from build123d import *

# Parameters (mm, degrees)
SKETCH_2_R          = 2.5
SKETCH_2_R_2        = 4
EXTRUDE_1_DEPTH     = 3
SKETCH_2_3_R        = 4
SKETCH_2_3_R_2      = 2
EXTRUDE_2_DEPTH     = 11.5
SKETCH_6_R          = 2
EXTRUDE_3_DEPTH     = 2.3
FILLET_1_R          = 2
SKETCH_7_R          = 2.5
SKETCH_7_R_2        = 2
CUT_EXTRUDE_2_DEPTH = 2
FILLET_2_R          = 1
CUT_EXTRUDE_3_REACH = 51.374
SKETCH_8_R          = 1.5
CUT_EXTRUDE_4_REACH = 51.374
SKETCH_11_R         = 1.5


with BuildPart() as part:
    # Sketch 2 → Extrude 1 (new body)
    with BuildSketch(Plane.XY):
        Polygon((-41.138288377, 15.425110404), (-41.138288377, 21.570131373), (-25.053133429, 21.570131373), (-20.677655191, 25.94560961), (-13.728698976, 25.94560961), (-8.574109119, 23.757870491), (35.231937864, 23.757870491), (41.138288377, 21.251065018), (41.138288377, -25.94560961), (-41.138288377, -25.94560961), (-41.138288377, -12.020899542), (-33.095710903, -12.020899542), (-33.095710903, 11.403821667), (-37.11699964, 11.403821667), align=None)
        with Locations((10.421946091, 8.532959579)):
            Circle(SKETCH_2_R, mode=Mode.SUBTRACT)
        with Locations((-7.306059133, -18.107570273)):
            Circle(SKETCH_2_R, mode=Mode.SUBTRACT)
        with Locations((25.421946091, 18.532959579)):
            Circle(SKETCH_2_R_2, mode=Mode.SUBTRACT)
        with Locations((-28.314407571, 7.976729123)):
            Circle(SKETCH_2_R_2, mode=Mode.SUBTRACT)
        with Locations((-17, 20.7)):
            Circle(SKETCH_2_R, mode=Mode.SUBTRACT)
        with BuildLine():
            Line((25.543402205, -5.467040421), (31.421946091, -5.467040421))
            ThreePointArc((31.421946091, -5.467040421), (32.129052872, -5.174147202), (32.421946091, -4.467040421))
            Line((32.421946091, -4.467040421), (32.421946091, 1.411503465))
            ThreePointArc((32.421946091, 1.411503465), (32.076213917, 2.167766389), (31.278078869, 2.401100465))
            ThreePointArc((31.278078869, 2.401100465), (26.799843583, 0.155062087), (24.553805205, -4.323173199))
            ThreePointArc((24.553805205, -4.323173199), (24.78713928, -5.121308248), (25.543402205, -5.467040421))
        make_face(mode=Mode.SUBTRACT)
    extrude(amount=EXTRUDE_1_DEPTH)

    # Sketch 2_3 → Extrude 2 (add)
    # profile 1 of 3: a face of its own
    with BuildSketch(Plane.XY):
        with Locations((-28.314407571, 7.976729123)):
            Circle(SKETCH_2_3_R)
        with Locations((-28.314407571, 7.976729123)):
            Circle(SKETCH_2_3_R_2, mode=Mode.SUBTRACT)
    # profile 2 of 3: a face of its own
    with BuildSketch(Plane.XY):
        with Locations((25.421946091, 18.532959579)):
            Circle(SKETCH_2_3_R)
        with Locations((25.421946091, 18.532959579)):
            Circle(SKETCH_2_3_R_2, mode=Mode.SUBTRACT)
    # profile 3 of 3: a face of its own
    with BuildSketch(Plane.XY):
        with BuildLine():
            Line((25.543402205, -5.467040421), (31.421946091, -5.467040421))
            ThreePointArc((31.421946091, -5.467040421), (32.129052872, -5.174147202), (32.421946091, -4.467040421))
            Line((32.421946091, -4.467040421), (32.421946091, 1.411503465))
            ThreePointArc((32.421946091, 1.411503465), (32.076213917, 2.167766389), (31.278078869, 2.401100465))
            ThreePointArc((31.278078869, 2.401100465), (26.799843583, 0.155062087), (24.553805205, -4.323173199))
            ThreePointArc((24.553805205, -4.323173199), (24.78713928, -5.121308248), (25.543402205, -5.467040421))
        make_face()
        with Locations((29.464448227, -2.509542558)):
            Circle(SKETCH_2_3_R_2, mode=Mode.SUBTRACT)
    extrude(amount=EXTRUDE_2_DEPTH)

    # Sketch 6 → Extrude 3 (add, symmetric)
    with BuildSketch(Plane(origin=(1.480786333, -5.526369829, 0), x_dir=(0, 0, 1), z_dir=(-0.25881904510252574, 0.9659258262890671, 0))):
        with Locations(Location((7.25, 26.715994864, 0), (0, 0, 90))):
            Circle(SKETCH_6_R)
    extrude(amount=EXTRUDE_3_DEPTH, both=True)

    # Fillet 1
    fillet_1_edges = [part.edges().sort_by_distance(p)[0] for p in [
        (24.75932029, 3.092229761, 7.25),
    ]]
    fillet(fillet_1_edges, radius=FILLET_1_R)

    # Sketch 7 → Cut-Extrude 2 (cut)
    with BuildSketch(Plane(origin=(1.480786333, -5.526369829, 0), x_dir=(0, 0, 1), z_dir=(-0.25881904510252574, 0.9659258262890671, 0))):
        with Locations((7.25, 26.715994864)):
            Circle(SKETCH_7_R)
        with Locations(Location((7.25, 26.715994864, 0), (0, 0, 270))):
            Circle(SKETCH_7_R_2, mode=Mode.SUBTRACT)
    extrude(amount=-CUT_EXTRUDE_2_DEPTH, mode=Mode.SUBTRACT)

    # Fillet 2
    fillet_2_edges = [part.edges().sort_by_distance(p)[0] for p in [
        (32.421946091, -1.527768478, 3),
        (32.129052872, -5.174147202, 3),
        (21.421946091, 18.532959579, 3),
        (-32.314407571, 7.976729123, 3),
        (28.482674148, -5.467040421, 3),
        (24.78713928, -5.121308248, 3),
        (26.799843583, 0.155062087, 3),
        (32.076213917, 2.167766389, 3),
    ]]
    fillet(fillet_2_edges, radius=FILLET_2_R)

    # Sketch 8 → Cut-Extrude 3 (cut, up to next)
    with BuildSketch(Plane.XY.offset(3), mode=Mode.PRIVATE) as cut_extrude_3_sk1:
        with Locations((-37.138288377, -18.983254576)):
            Circle(SKETCH_8_R)
    cut_extrude_3_tool1 = extrude(cut_extrude_3_sk1.sketch, amount=-CUT_EXTRUDE_3_REACH, mode=Mode.PRIVATE) & part.part
    # Sketch 8 → Cut-Extrude 3 (cut, up to next)
    with BuildSketch(Plane.XY.offset(3), mode=Mode.PRIVATE) as cut_extrude_3_sk2:
        with Locations((-31.138288377, -18.983254576)):
            Circle(SKETCH_8_R)
    cut_extrude_3_tool2 = extrude(cut_extrude_3_sk2.sketch, amount=-CUT_EXTRUDE_3_REACH, mode=Mode.PRIVATE) & part.part
    add(cut_extrude_3_tool1.solids().sort_by_distance((-37.138288, -18.983255, 3))[0], mode=Mode.SUBTRACT)
    add(cut_extrude_3_tool2.solids().sort_by_distance((-31.138288, -18.983255, 3))[0], mode=Mode.SUBTRACT)

    # Sketch 11 → Cut-Extrude 4 (cut, up to next)
    with BuildSketch(Plane.XY.offset(3), mode=Mode.PRIVATE) as cut_extrude_4_sk1:
        with Locations((37.138288377, -18.983254576)):
            Circle(SKETCH_11_R)
    cut_extrude_4_tool1 = extrude(cut_extrude_4_sk1.sketch, amount=-CUT_EXTRUDE_4_REACH, mode=Mode.PRIVATE) & part.part
    # Sketch 11 → Cut-Extrude 4 (cut, up to next)
    with BuildSketch(Plane.XY.offset(3), mode=Mode.PRIVATE) as cut_extrude_4_sk2:
        with Locations((31.138288377, -18.983254576)):
            Circle(SKETCH_11_R)
    cut_extrude_4_tool2 = extrude(cut_extrude_4_sk2.sketch, amount=-CUT_EXTRUDE_4_REACH, mode=Mode.PRIVATE) & part.part
    add(cut_extrude_4_tool1.solids().sort_by_distance((37.138288, -18.983255, 3))[0], mode=Mode.SUBTRACT)
    add(cut_extrude_4_tool2.solids().sort_by_distance((31.138288, -18.983255, 3))[0], mode=Mode.SUBTRACT)


solid = part.part
Read the model definition and answer for the solid it produces. Units are mm, in the model's axes. A direction names the side the tool comes from. Coordinates: 2 decimals unless noted, no trailing zeros. Write each loop counter-clockwise with the first axis right and the second up, starting at its lowest first coordinate (ties: lowest second). Pieces come first, ordered by that corner, then holes. Notation, with made-up numbers: M 17.5,87.25 L 73.5,87.25 A26 cw 73.5,107.25 Z; hole C 21.25,73.25 d8. An arc over 180 degrees is marked long. Use a Markdown table: item, result.
Q1. Determine the mould class of faces 4 (the face through (32.524, -19.558, 1.521)), 5 (the face through (-33, 21.57, 1)), 6 (the face through (27.3, 15, 7.7)) for opening direction X: released by +X, released by -X, zero draft, split by the parting line, or undercut.
Answer block:
| item | result |
|---|---|
| face 4 | undercut |
| face 5 | zero draft |
| face 6 | split by the parting line |
Q2. Which of the six approach directions +Z, -Z, +X, -X, +Y, -Y give full straight-line access (tool end or side, diameter ignored) to faces 1 (the face through (32.422, -2, 8)), 2 (the face through (-32.31, 8.15, 7.68)), 3 (the face through (28, -5.467, 8))?
Answer block:
| item | result |
|---|---|
| face 1 | +Z, +X, +Y, -Y |
| face 2 | +Z |
| face 3 | +Z, +X, -X, -Y |
Q3. The part is cut by section C-C, the plane x = 4. Write down the section's boundary in (y, z).
Answer block:
| item | result |
|---|---|
| outline | M -25.95,0 L 23.76,0 L 23.76,3 L -25.95,3 Z |
Q4. Straight lines are drawn through the part: L1, parallel to Z at x = -16.5, y = -14.5; L2, parallel to X at y = 1, z = 9; L3, parallel to Y at x = 25, z = 1.5. For each, find the intervals that lie inside material, in ascending order. Write a range as [from, to].
Answer block:
| item | result |
|---|---|
| L1 | z = [0, 3] |
| L2 | x = [26.39, 28.39], [29.24, 32.42] |
| L3 | y = [-25.95, 16.58], [20.49, 23.76] |
Q5. The part is cut by section B-B, the plane y = -16.5. Write down the section's boundary in (x, z).
Answer block:
| item | result |
|---|---|
| outline | M -41.14,0 L -9.22,0 L -9.22,3 L -41.14,3 Z; M -5.39,0 L 41.14,0 L 41.14,3 L -5.39,3 Z |
Q6. Each of these flat-tipped pins is pushed along its axis until it touches: pin 1 Ø3.5 at (x, y) = (-31.14, -18.98) entering from +Z; pin 2 Ø3.5 at (x, z) = (8.5, 2) entering from +Y; pin 3 Ø3.5 at (x, y) = (-28.31, 7.98) entering from +Z; pin 4 Ø3.5 at (y, z) = (2, 2) entering from -X. Where does it stop, or does it pass through?
Answer block:
| item | result |
|---|---|
| pin 1 | stops at z = 3 |
| pin 2 | stops at y = 23.76 |
| pin 3 | passes through |
| pin 4 | stops at x = -33.1 |
Q7. The part is cut by section A-A, the plane x = -15.5. Write down the section's boundary in (y, z), then the cut area to 3 significant figures.
Answer block:
| item | result |
|---|---|
| outline | M -25.95,0 L 18.7,0 L 18.7,3 L -25.95,3 Z; M 22.7,0 L 25.95,0 L 25.95,3 L 22.7,3 Z |
| area | 144 mm2 |
